Source: three-view drawing plus pictorial views. Frame: mm from the lowest corner of the part. Give positions to 0.01 mm unless a question says otherwise; leave off trailing zeros. Loops run counter-clockwise (first coordinate to the right, second up) from the corner with the lowest first, then second, coordinate; pieces in that order, holes last. Notation, with made-up numbers: M 26.5,15.25 L 68.5,15.25 A17 cw 68.5,45.25 Z; hole C 50,12 d9. An arc over 180 degrees is marked long. Write item = value, one per line.
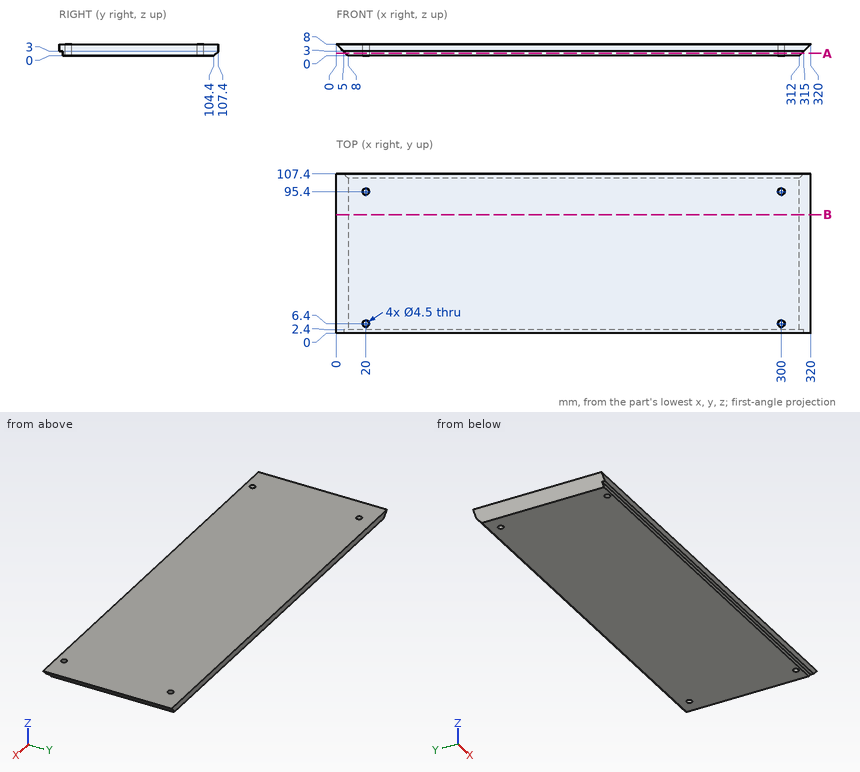
1. First-contact query: pin 1 Ø0.9 at (x, z) = (161.5, 2) entering from -Y; pin 2 Ø5 at (x, y) = (20, 6.4) entering from +Z; pin 3 Ø1 at (y, z) = (53.5, 5) entering from -X; pin 4 Ø2 at (y, z) = (82.5, 2) entering from -X. Flat tips, straight axial feed; report the tip coordinate or a pass-through.
Derived:
pin_1 = 2.4
pin_2 = 8
pin_3 = 2.5
pin_4 = 5
2. Cut plane A-A, the plane z = 1.75. Return the cut outline in (x, y), then the cut area to 3 significant figures.
Derived:
outline = M 6.25,2.4 L 313.75,2.4 L 313.75,106.15 L 6.25,106.15 Z; hole C 20,6.4 d4.5; hole C 20,95.4 d4.5; hole C 300,6.4 d4.5; hole C 300,95.4 d4.5
area = 31,800 mm²
3. Cut plane B-B, the plane y = 80. Return the cut outline in (x, z), then the cut area to 3 significant figures.
Derived:
outline = M 0,8 L 8,0 L 312,0 L 320,8 Z
area = 2,500 mm²
4. Material intervals for probe 1 along Y at (x, z) = (20, 6.65); probe 2 along Y at (x, z) = (20, 1.5); probe 3 along X at (y, z) = (95.4, 2.05), sorted ascending. Write a range as from..to.
Derived:
probe_1 = 0..4.15, 8.65..93.15, 97.65..107.4
probe_2 = 2.4..4.15, 8.65..93.15, 97.65..105.9
probe_3 = 5.95..17.75, 22.25..297.75, 302.25..314.05
